from build123d import *

# Parameters (mm, degrees)
SKETCH_1_W          = 75
SKETCH_1_H          = 61
EXTRUDE_1_DEPTH     = 2
SKETCH_2_W          = 28
SKETCH_2_H          = 11
CUT_EXTRUDE_1_DEPTH = 97.695398029
SKETCH_3_W          = 10
SKETCH_3_H          = 5
SKETCH_3_W_2        = 8
SKETCH_3_H_2        = 8
CUT_EXTRUDE_2_DEPTH = 97.695398029
SKETCH_4_R          = 1.35
CUT_EXTRUDE_3_DEPTH = 97.695398029
SKETCH_5_R          = 2
CUT_EXTRUDE_4_DEPTH = 97.695398029


with BuildPart() as part:
    # 草图1 → 凸台-拉伸1 (new body)
    with BuildSketch(Plane.XY):
        with Locations((37.5, 30.5)):
            Rectangle(SKETCH_1_W, SKETCH_1_H)
    extrude(amount=EXTRUDE_1_DEPTH)

    # 草图2 → 切除-拉伸1 (cut, through all)
    with BuildSketch(Plane.XY):
        with Locations((53.5, 9.4)):
            Rectangle(SKETCH_2_W, SKETCH_2_H)
    extrude(amount=CUT_EXTRUDE_1_DEPTH, mode=Mode.SUBTRACT)

    # 草图3 → 切除-拉伸2 (cut, through all)
    with BuildSketch(Plane.XY):
        with Locations((37.5, 51)):
            Rectangle(SKETCH_3_W, SKETCH_3_H)
        with Locations((60.5, 42)):
            Rectangle(SKETCH_3_W_2, SKETCH_3_H_2)
    extrude(amount=CUT_EXTRUDE_2_DEPTH, mode=Mode.SUBTRACT)

    # 草图4 → 切除-拉伸3 (cut, through all)
    with BuildSketch(Plane.XY):
        with Locations((6.5, 18)):
            Circle(SKETCH_4_R)
        with Locations((68.5, 18)):
            Circle(SKETCH_4_R)
        with Locations((6.5, 54)):
            Circle(SKETCH_4_R)
        with Locations((68.5, 54)):
            Circle(SKETCH_4_R)
    extrude(amount=CUT_EXTRUDE_3_DEPTH, mode=Mode.SUBTRACT)

    # 草图5 → 切除-拉伸4 (cut, through all)
    with BuildSketch(Plane.XY):
        with Locations((17.5, 50)):
            Circle(SKETCH_5_R)
    extrude(amount=CUT_EXTRUDE_4_DEPTH, mode=Mode.SUBTRACT)


solid = part.part
Can you work these out from the model? Positions are in its coordinate system, mm. A direction names the side the tool comes from. Give positions to 0.01 mm unless a question says otherwise; leave off trailing zeros. Order: outer loops, then holes, each group sorted by start corner. A loop starts at its lowest first (then second) coordinate and runs counter-clockwise, first axis right, second up. Notation, with made-up numbers: (44, -16.5) - (59, -16.5) arc R23 ccw to (59, 16.5) - close; hole circle Ø7 at (-36, 6). An arc over 180 degrees is marked (long way). Write each question's results on one line, items separated by ' | '.
1) On a 3-axis mill with a long thin cutter (end or side, diameter ignored), from which of +Z, -Z, +X, -X, +Y, -Y can I reach the whole of each face in a straight line? I mean faces 5 (the face through (60, 38, 1)), 6 (the face through (37, 31, 0)). Say none if no direction works.
Final values:
face 5: +Z, -Z | face 6: -Z, +X, -X, +Y, -Y
2) Suppose I cut it at B-B, the plane z = 1.6. Give the number of separate pieces and of enclosed holes in the cut face, then the cut area to 3 significant figures.
Final values:
separate pieces: 1 | enclosed holes: 8 | area: 4,120 mm^2
3) Suppose I cut it at D-D, the plane x = 47. Write out the boundary of the cut face in (y, z), then the cut area to 3 significant figures.
Final values:
outline: (0, 0) - (3.9, 0) - (3.9, 2) - (0, 2) - close; (14.9, 0) - (61, 0) - (61, 2) - (14.9, 2) - close | area: 100 mm^2
4) Please list where these lines run through material, in increasing order: line 1 along X through (y, z) = (54, 0.6); line 2 along Y through (x, z) = (68.5, 1.15); line 3 along X through (y, z) = (50, 0.45). Write a range as [from, to].
Final values:
line 1: x = [0, 5.15], [7.85, 67.15], [69.85, 75] | line 2: y = [0, 16.65], [19.35, 52.65], [55.35, 61] | line 3: x = [0, 15.5], [19.5, 32.5], [42.5, 75]
5) If we mould it in two halves opening along X, with no side actions, what happens to faces 1 (the face through (0, 30, 1)), 2 (the face through (42.5, 51, 1)), 3 (the face through (37, 0, 1)), 4 (the face through (69.747, 17.483, 0.986))? For each: pulls with the +X half, pulls with the -X half, needs draft (parallel to the pull), parting line crosses it, or undercut.
Final values:
face 1: pulls with the -X half | face 2: undercut | face 3: needs draft | face 4: undercut
6) Suppose I cut it at C-C, the plane x = 68.5. Write out the boundary of the cut face in (y, z).
Final values:
outline: (0, 0) - (16.65, 0) - (16.65, 2) - (0, 2) - close; (19.35, 0) - (52.65, 0) - (52.65, 2) - (19.35, 2) - close; (55.35, 0) - (61, 0) - (61, 2) - (55.35, 2) - close
7) Suppose I cut it at A-A, the plane y = 50. Write out the boundary of the cut face in (x, z).
Final values:
outline: (0, 0) - (15.5, 0) - (15.5, 2) - (0, 2) - close; (19.5, 0) - (32.5, 0) - (32.5, 2) - (19.5, 2) - close; (42.5, 0) - (75, 0) - (75, 2) - (42.5, 2) - close
